The drawing under review shows one solid part. Ordinate dimensions are in mm from its lowest x, y, z. A direction names the side the tool comes from. Round coordinates to 2 decimals unless told otherwise and drop trailing zeros. Order: outer loops, then holes, each group sorted by start corner. A loop starts at its lowest first (then second) coordinate and runs counter-clockwise, first axis right, second up. Notation, with made-up numbers: (32.25, 78.5) - (39.25, 78.5) arc R22 cw to (39.25, 105.5) - close; hole circle Ø5 at (55.25, 88). An arc over 180 degrees is marked (long way). One line per question, with ' | ' between items.
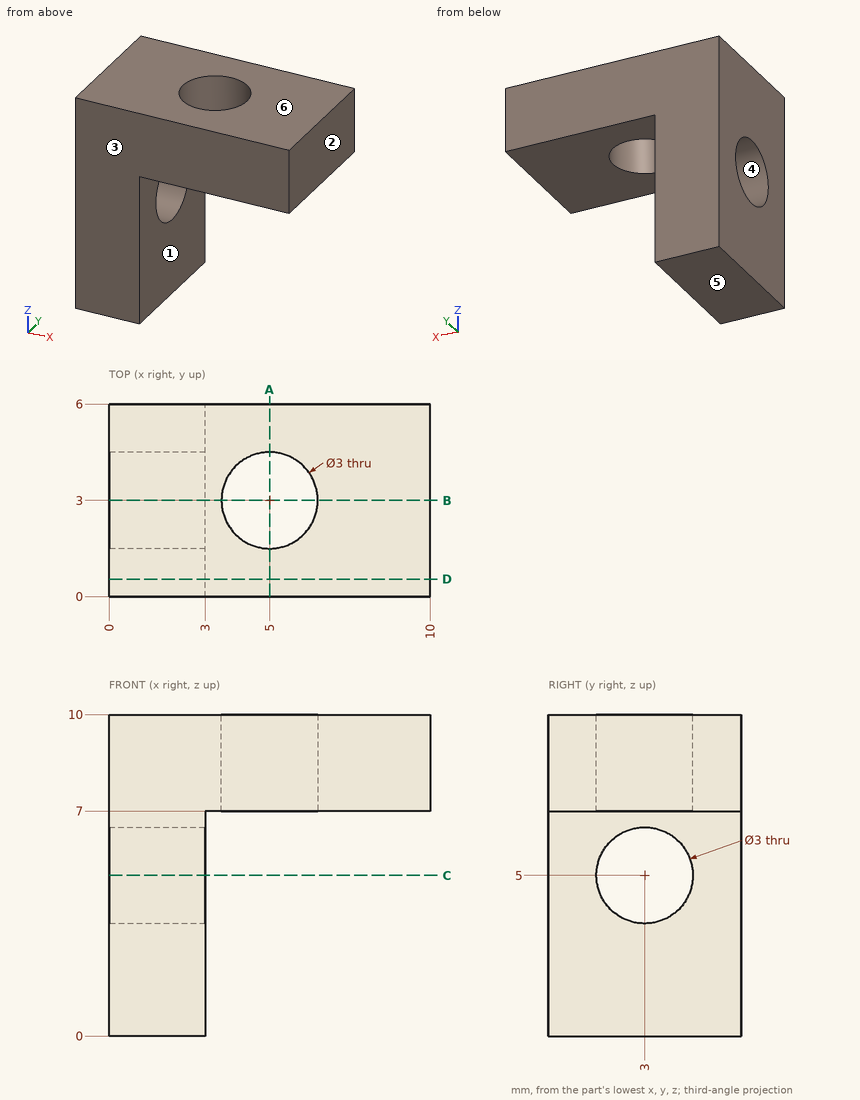
(1) We need section B-B on y = 3. State the section outline as (x, z) points, plus the area to 3 significant figures.
Output values:
outline: (0, 0) - (3, 0) - (3, 3.5) - (0, 3.5) - close; (0, 6.5) - (3, 6.5) - (3, 7) - (3.5, 7) - (3.5, 10) - (0, 10) - close; (6.5, 7) - (10, 7) - (10, 10) - (6.5, 10) - close | area: 33.0 mm^2
(2) Mouldability with a two-part tool opening along Z and no side actions: class the marked faces 3, 4, 5 and 6 as released by +Z, released by -Z, zero draft, split by the parting line, or undercut.
Output values:
face 3: zero draft | face 4: undercut | face 5: released by -Z | face 6: released by +Z
(3) For probe 1 along Y at (x, z) = (5, 9); probe 2 along Z at (x, y) = (4.75, 5.6); probe 3 along X at (y, z) = (1.05, 1.5), list the stretches that pass through material, from the lowest coordinate up. Write a range as [from, to].
Output values:
probe 1: [0, 1.5], [4.5, 6] | probe 2: [7, 10] | probe 3: [0, 3]
(4) We need section A-A on x = 5. State the section outline as (y, z) points, plus the area to 3 significant figures.
Output values:
outline: (0, 7) - (1.5, 7) - (1.5, 10) - (0, 10) - close; (4.5, 7) - (6, 7) - (6, 10) - (4.5, 10) - close | area: 9.00 mm^2
(5) For the marked faces 1 and 2, list the 3-axis set-ups (+Z, -Z, +X, -X, +Y, -Y) from which the entire face can be reached by the end or side of a thin tool; tool diameter is ignored.
Output values:
face 1: -Z, +X, +Y, -Y | face 2: +Z, -Z, +X, +Y, -Y
(6) We need section C-C on z = 5. State the section outline as (x, y) points, plus the area to 3 significant figures.
Output values:
outline: (0, 0) - (3, 0) - (3, 1.5) - (0, 1.5) - close; (0, 4.5) - (3, 4.5) - (3, 6) - (0, 6) - close | area: 9.00 mm^2
(7) We need section D-D on y = 0.55. State the section outline as (x, z) points.
Output values:
outline: (0, 0) - (3, 0) - (3, 7) - (10, 7) - (10, 10) - (0, 10) - close
(8) Insertion check: pin 1 (2.5 mm diameter, centred on y = 3, z = 5, fed in from -X); pin 2 (1.5 mm diameter, centred on y = 4.5, z = 6, fed in from +X); pin 3 (3 mm diameter, centred on x = 6, y = 2.5, fed in from -Z). Each pin has a flat end and moves straight along its axis. Give the tip position at first contact, or say it passes through.
Output values:
pin 1: through | pin 2: x = 3 | pin 3: z = 7
